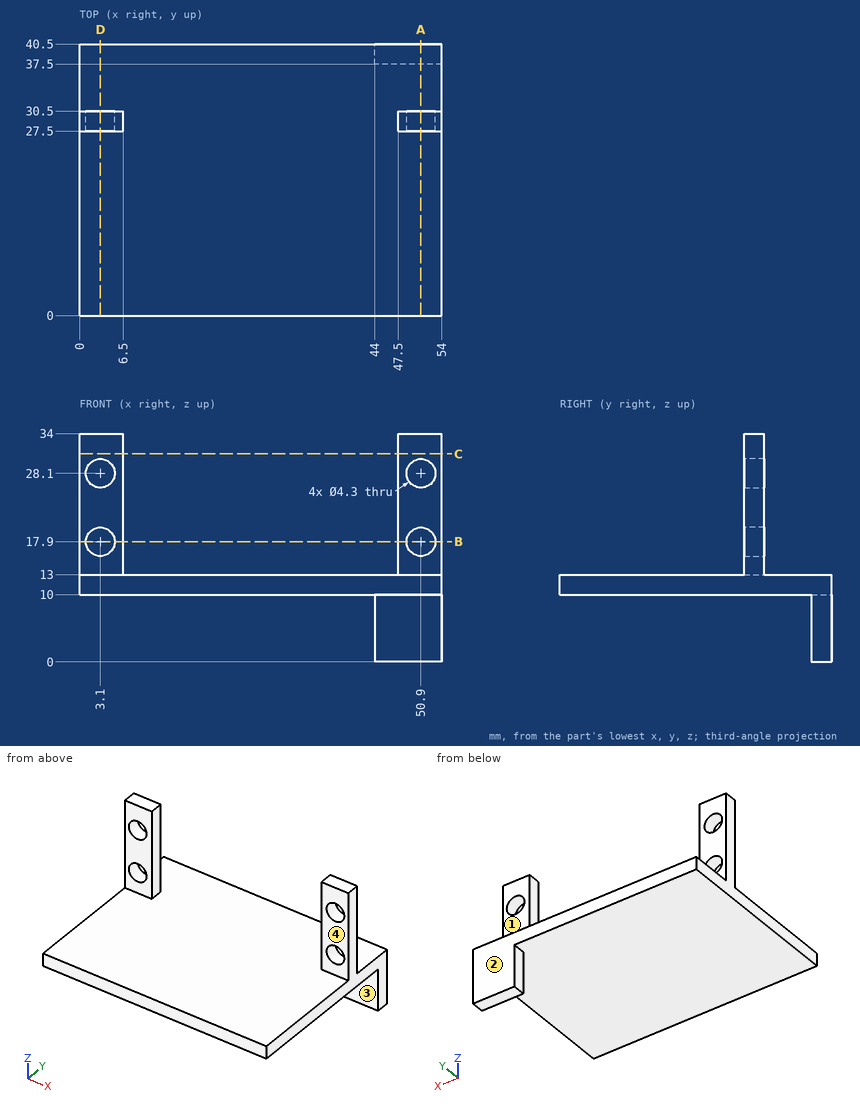
Answer from the drawing. Dimensions are ordinates in mm from the lowest x, y and z of the part. A direction names the side the tool comes from. Round coordinates to 2 decimals unless told otherwise and drop trailing zeros. Write each loop counter-clockwise with the first axis right and the second up, starting at its lowest first coordinate (ties: lowest second). Pieces come first, ordered by that corner, then holes. Notation, with made-up numbers: M 89.5,-32 L 131.5,-32 A14 cw 131.5,-5 Z; hole C 89.5,84 d10. An arc over 180 degrees is marked long. Write each question's results on one line, items separated by ' | '. Start each with the question number.
Item 1: For the marked faces 1, 2, 3 and 4, determine the directions among +Z, -Z, +X, -X, +Y, -Y from which every point of the face is accessible in a straight line to the end or side of a thin tool.
Item 2: A cutting plane is placed at D-D on x = 3.1. Write down the section's boundary in (y, z), and give its area (3 significant figures).
Item 3: A cutting plane is placed at A-A on x = 50.9. Write down the section's boundary in (y, z), and give its area (3 significant figures).
Item 4: Straight lines are drawn through the part: L1, parallel to X at y = 28.2, z = 17.9; L2, parallel to Z at x = 50, y = 29; L3, parallel to Z at x = 8.5, y = 19. For each, find the intervals that lie inside material, in ascending order. Write a range as [from, to].
Item 5: Flat-ended cylindrical pins translate along their axes: pin 1 Ø8 at (x, z) = (47.5, 3) entering from -Y; pin 2 Ø2 at (x, z) = (50.5, 23) entering from -Y; pin 3 Ø4 at (x, y) = (38, 12.5) entering from +Z; pin 4 Ø1.5 at (y, z) = (29, 26.5) entering from -X. Find the tip coordinate at first contact, or state that the pin passes through.
Item 6: A cutting plane is placed at B-B on z = 17.9. Write down the section's boundary in (x, y).
Item 7: A cutting plane is placed at C-C on z = 31. Write down the section's boundary in (x, y).
Check sheet entries:
1) face 1: +Z, +X, -X, +Y | face 2: +Z, -Z, +X, -X, +Y | face 3: -Z, +X, -X, -Y | face 4: +Z, +X, -X, -Y
2) outline: M 0,10 L 40.5,10 L 40.5,13 L 30.5,13 L 30.5,15.75 L 27.5,15.75 L 27.5,13 L 0,13 Z; M 27.5,20.05 L 30.5,20.05 L 30.5,25.95 L 27.5,25.95 Z; M 27.5,30.25 L 30.5,30.25 L 30.5,34 L 27.5,34 Z | area: 159 mm²
3) outline: M 0,10 L 37.5,10 L 37.5,0 L 40.5,0 L 40.5,13 L 30.5,13 L 30.5,15.75 L 27.5,15.75 L 27.5,13 L 0,13 Z; M 27.5,20.05 L 30.5,20.05 L 30.5,25.95 L 27.5,25.95 Z; M 27.5,30.25 L 30.5,30.25 L 30.5,34 L 27.5,34 Z | area: 189 mm²
4) L1: [0, 0.95], [5.25, 6.5], [47.5, 48.75], [53.05, 54] | L2: [10, 15.95], [19.85, 26.15], [30.05, 34] | L3: [10, 13]
5) pin 1: y = 37.5 | pin 2: y = 27.5 | pin 3: z = 13 | pin 4: x = 0
6) outline: M 0,27.5 L 0.95,27.5 L 0.95,30.5 L 0,30.5 Z; M 5.25,27.5 L 6.5,27.5 L 6.5,30.5 L 5.25,30.5 Z; M 47.5,27.5 L 48.75,27.5 L 48.75,30.5 L 47.5,30.5 Z; M 53.05,27.5 L 54,27.5 L 54,30.5 L 53.05,30.5 Z
7) outline: M 0,27.5 L 6.5,27.5 L 6.5,30.5 L 0,30.5 Z; M 47.5,27.5 L 54,27.5 L 54,30.5 L 47.5,30.5 Z
